Geometry: final body of the model. Coordinates: model frame, mm. Give positions to 0.01 mm unless a question says otherwise; leave off trailing zeros. Write each loop counter-clockwise with the first axis right and the second up, starting at its lowest first coordinate (ties: lowest second). Pieces come first, ordered by that corner, then holes. Notation, with made-up numbers: (86.25, 81.5) -> (109.25, 81.5) arc R11 ccw to (109.25, 88.5) -> close; hole circle Ø11 at (-16, -18). An arc over 180 degrees is marked (long way). Answer as a JSON object with one key per item and string values.
from build123d import *

# Parameters (mm, degrees)
ESQUISSE3_W        = 200
ESQUISSE3_H        = 200
ESQUISSE3_R        = 5
BOSS_EXTRU_2_DEPTH = 7
CONG_1_R           = 15


with BuildPart() as part:
    # Esquisse3 → Boss.-Extru.2 (new body)
    with BuildSketch(Plane.XY):
        Rectangle(ESQUISSE3_W, ESQUISSE3_H)
        with Locations((80, 80)):
            Circle(ESQUISSE3_R, mode=Mode.SUBTRACT)
        with Locations((80, -80)):
            Circle(ESQUISSE3_R, mode=Mode.SUBTRACT)
        with Locations((-80, -80)):
            Circle(ESQUISSE3_R, mode=Mode.SUBTRACT)
        with Locations((-80, 80)):
            Circle(ESQUISSE3_R, mode=Mode.SUBTRACT)
    extrude(amount=BOSS_EXTRU_2_DEPTH)

    # Congé1
    cong_1_edges = [part.edges().sort_by_distance(p)[0] for p in [
        (-100, 100, 3.5),
        (100, 100, 3.5),
        (100, -100, 3.5),
        (-100, -100, 3.5),
    ]]
    fillet(cong_1_edges, radius=CONG_1_R)


solid = part.part
Q1. First-contact query: P1, Ø6, axis at x = -80, y = -80, coming from the -Z side. Flat tip, straight axial feed; report the tip coordinate or a pass-through.
Values:
{"P1": "through"}
Q2. Material intervals for L1, parallel to Y at x = -80, z = 3.5; L2, parallel to X at y = 78, z = 5.75; L3, parallel to X at y = 83, z = 6.25, sorted ascending. Write a range as from..to.
Values:
{"L1": "-100..-85, -75..75, 85..100", "L2": "-100..-84.58, -75.42..75.42, 84.58..100", "L3": "-100..-84, -76..76, 84..100"}
Q3. Mould query, pull axis Y, two halves, no side actions, for faces 1 (the cylindrical face through (-95.72, -95.49, 3.55)), 2 (the cylindrical face through (84.619, -81.915, 3.451)), 3 (the flat face through (100, -1, 3)). Classes: pulls with the +Y half, pulls with the -Y half, needs draft (parallel to the pull), parting line crosses it, or undercut.
Values:
{"face 1": "pulls with the -Y half", "face 2": "undercut", "face 3": "needs draft"}
Q4. Cut plane A-A (x = -80). Return the cut outline in (y, z).
Values:
{"outline": "(-100, 0) -> (-85, 0) -> (-85, 7) -> (-100, 7) -> close; (-75, 0) -> (75, 0) -> (75, 7) -> (-75, 7) -> close; (85, 0) -> (100, 0) -> (100, 7) -> (85, 7) -> close"}
